Verification items for the finished model (mm, model axes). A direction names the side the tool comes from. Give positions to 0.01 mm unless a question says otherwise; leave off trailing zeros. Loops run counter-clockwise (first coordinate to the right, second up) from the corner with the lowest first, then second, coordinate; pieces in that order, holes last. Notation, with made-up numbers: (16, 44.25) - (55, 44.25) arc R6 ccw to (55, 55.25) - close; hole circle Ø3 at (16.25, -31.75). An arc over 180 degrees is marked (long way). Put each result on its own line as item: value. Start each with the question number.
```python
from build123d import *

# Parameters (mm, degrees)
SKETCH1_R                   = 6
ARM_INSERT_DEPTH            = 30
SKETCH2_W                   = 14
SKETCH2_H                   = 14
FACE_PLATE_DEPTH            = 3
SKETCH3_R                   = 2
SKETCH3_R_2                 = 2.5
MOTOR_MOUNT_DEPTH           = 3
MOTOR_MOUNT_SUPPORT_1_DEPTH = 2.5
MOTOR_MOUNT_SUPPORT_2_DEPTH = 2.5
SKETCH8_R                   = 2.5
LIGHTENING_HOLE_DEPTH       = 68.841325022


with BuildPart() as part:
    # Sketch1 → Arm Insert (new body)
    with BuildSketch(Plane.XY):
        Circle(SKETCH1_R)
    extrude(amount=ARM_INSERT_DEPTH)

    # Sketch2 → Face Plate (add)
    with BuildSketch(Plane.XY.offset(30)):
        Rectangle(SKETCH2_W, SKETCH2_H)
    extrude(amount=FACE_PLATE_DEPTH)

    # Sketch3 → Motor Mount (add)
    # profile 1 of 2: a face of its own
    with BuildSketch(Plane(origin=(0, 7, 0), x_dir=(1, 0, 0), z_dir=(0, 1, 0))):
        with BuildLine():
            ThreePointArc((-7, -30.935385736), (-7.206551185, -32.957355148), (-7.817672061, -34.895796524))
            Line((-7.817672061, -34.895796524), (-12.803400836, -46.455354126))
            ThreePointArc((-12.803400836, -46.455354126), (0.006350978, -38.000003191), (12.870800409, -46.371899141))
            Line((12.870800409, -46.371899141), (7.843612764, -34.921493496))
            ThreePointArc((7.843612764, -34.921493496), (7.213175378, -32.95526455), (7, -30.901472004))
            Line((7, -30.901472004), (7, -33))
            Line((7, -33), (-7, -33))
            Line((-7, -33), (-7, -30.935385736))
        make_face()
    # profile 2 of 2: a face of its own
    with BuildSketch(Plane(origin=(0, 7, 0), x_dir=(1, 0, 0), z_dir=(0, 1, 0))):
        with BuildLine():
            ThreePointArc((12.870800409, -46.371899141), (0.006350978, -38.000003191), (-12.803400836, -46.455354126))
            ThreePointArc((-12.803400836, -46.455354126), (-2.778898897, -65.710757571), (14.051858279, -51.999929229))
            ThreePointArc((14.051858279, -51.999929229), (13.75341275, -49.124619665), (12.870800409, -46.371899141))
        make_face()
        with Locations(Location((-9.448141721, -51.999929229, 0), (0, 0, 270))):
            Circle(SKETCH3_R, mode=Mode.SUBTRACT)
        with Locations(Location((0.051858279, -59.999929229, 0), (0, 0, 270))):
            Circle(SKETCH3_R, mode=Mode.SUBTRACT)
        with Locations(Location((0.051858279, -51.999929229, 0), (0, 0, 270))):
            Circle(SKETCH3_R_2, mode=Mode.SUBTRACT)
        with Locations(Location((9.551858279, -51.999929229, 0), (0, 0, 270))):
            Circle(SKETCH3_R, mode=Mode.SUBTRACT)
        with Locations(Location((0.051858279, -43.999929229, 0), (0, 0, 270))):
            Circle(SKETCH3_R, mode=Mode.SUBTRACT)
    extrude(amount=-MOTOR_MOUNT_DEPTH)

    # Sketch4 → Motor Mount Support 1 (add)
    with BuildSketch(Plane(origin=(6.098650662, 0, 2.630396348), x_dir=(-0.39604107883214285, 0, 0.9182327939457796), z_dir=(-0.9182327939457796, 0, -0.39604107883214285))):
        with BuildLine():
            Line((31.696620561, -7), (31.696620561, 4))
            Line((31.696620561, 4), (41.433043154, 4))
            add(Edge.make_bspline(
                [(41.433043154, 4), (31.696620561, 4), (31.696620561, -7)],
                knots=[3.141592654, 3.141592654, 3.141592654, 4.71238898, 4.71238898, 4.71238898], degree=2, weights=[1, 0.707106781, 1]))
        make_face()
    extrude(amount=-MOTOR_MOUNT_SUPPORT_1_DEPTH)

    # Sketch5 → Motor Mount Support 2 (add)
    with BuildSketch(Plane(origin=(-6.278168341, 0, 2.756367878), x_dir=(-0.402002149140903, 0, -0.9156387235619163), z_dir=(0.9156387235619163, 0, -0.402002149140903))):
        with BuildLine():
            Line((-31.656634836, -7), (-31.656634836, 4))
            Line((-31.656634836, 4), (-41.381308441, 4))
            add(Edge.make_bspline(
                [(-31.656634836, -7), (-31.656634836, 4), (-41.381308441, 4)],
                knots=[1.570796327, 1.570796327, 1.570796327, 3.141592654, 3.141592654, 3.141592654], degree=2, weights=[1, 0.707106781, 1]))
        make_face()
    extrude(amount=-MOTOR_MOUNT_SUPPORT_2_DEPTH)

    # Sketch8 → Lightening Hole (cut, through all)
    with BuildSketch(Plane(origin=(0, 0, 0), x_dir=(-1, 0, 0), z_dir=(0, 0, -1))):
        Circle(SKETCH8_R)
    extrude(amount=-LIGHTENING_HOLE_DEPTH, mode=Mode.SUBTRACT)


solid = part.part
```
1) Set-up check for faces 1 (the face through (-5.186, 1.715, 35.106)), 2 (the face through (-6, 0, 15)), 3 (the face through (-7, -2, 31)), 4 (the face through (7, -2, 31)): record each of +Z, -Z, +X, -X, +Y, -Y from which the full face is reachable in a straight line by a thin tool's end or side.
2) Section check C-C, the plane x = 3.5. Enter the section's corners in (y, z).
3) Scan lines: line 1 along X through (y, z) = (1.25, 17.5); line 2 along X through (y, z) = (1, 28); line 3 along Z through (x, y) = (3.75, 0). Record each from-to range of solid material in increasing order. Write a range as from..to.
4) Draft check along Z on faces 5 (the face through (7.22, 5.52, 32.98)), 6 (the face through (9.6, 5.5, 50)), 7 (the face through (5.19, 2, 35.1)). Enter one of: pulls with the +Z half, pulls with the -Z half, needs draft (parallel to the pull), parting line crosses it, or undercut.
5) Section check B-B, the plane z = 24. Enter the section's corners in (x, y).
6) Depth check by flat-ended pin: P1, Ø1, axis at x = -6, y = -3.5, coming from the +Z side; P2, Ø1.5, axis at y = 4, z = 45.5, coming from the +X side; P3, Ø8, axis at x = 0.05, z = 52, coming from the +Y side; P4, Ø14, axis at x = 7, z = 44.5, coming from the -Y side. Enter the tip coordinate at first touch or a pass-through.
7) Section check A-A, the plane z = 60.5. Enter the section's corners in (x, y).
Results are:
1. face 1: +Z, -Y
1. face 2: -Z
1. face 3: -Z, -X, -Y
1. face 4: -Z, +X, -Y
2. outline: (-7, 30) - (-4.87, 30) - (-4.87, 0) - (4.87, 0) - (4.87, 30) - (7, 30) - (7, 65.57) - (4, 65.57) - (4, 33) - (-7, 33) - close
3. line 1: x = -5.87..-2.17, 2.17..5.87
3. line 2: x = -5.92..-2.29, 2.29..5.92
3. line 3: z = 0..33
4. face 5: pulls with the -Z half
4. face 6: undercut
4. face 7: pulls with the +Z half
5. outline: circle Ø12 at (0, 0); hole circle Ø5 at (0, 0)
6. P1: stops at z = 33
6. P2: stops at x = 12.82
6. P3: stops at y = 7
6. P4: stops at y = 2.76
7. outline: (-11.07, 4) - (-1.88, 4) - (-1.88, 7) - (-11.07, 7) - close; (1.99, 4) - (11.18, 4) - (11.18, 7) - (1.99, 7) - close
